```python
from build123d import *

# Parameters (mm, degrees)
SKETCH_1_W          = 30
SKETCH_1_H          = 40
SKETCH_1_W_2        = 28
SKETCH_1_H_2        = 38
EXTRUDE_1_DEPTH     = 250
SKETCH_3_R          = 2.1
CUT_EXTRUDE_1_DEPTH = 250
SKETCH_4_R          = 3.5
CUT_EXTRUDE_2_DEPTH = 250
SKETCH_5_R          = 7
CUT_EXTRUDE_3_DEPTH = 250
CUT_EXTRUDE_4_DEPTH = 20
CUT_EXTRUDE_START   = -20
SKETCH_8_R          = 3.25
CUT_EXTRUDE_7_DEPTH = 22
SKETCH_9_R          = 2
CUT_EXTRUDE_8_DEPTH = 36


with BuildPart() as part:
    # 草图1 → 凸台-拉伸1 (new body)
    with BuildSketch(Plane.XY):
        Rectangle(SKETCH_1_W, SKETCH_1_H)
        Rectangle(SKETCH_1_W_2, SKETCH_1_H_2, mode=Mode.SUBTRACT)
    extrude(amount=EXTRUDE_1_DEPTH)

    # 草图3 → 切除-拉伸1 (cut)
    with BuildSketch(Plane(origin=(0, 20, 0), x_dir=(1, 0, 0), z_dir=(0, 1, 0))):
        with Locations(Location((5, -7.5, 0), (0, 0, 270))):
            Circle(SKETCH_3_R)
        with Locations(Location((5, -22.5, 0), (0, 0, 270))):
            Circle(SKETCH_3_R)
        with Locations(Location((5, -227.5, 0), (0, 0, 90))):
            Circle(SKETCH_3_R)
        with Locations(Location((5, -242.5, 0), (0, 0, 90))):
            Circle(SKETCH_3_R)
        with Locations(Location((0, -120, 0), (0, 0, 270))):
            Circle(SKETCH_3_R)
        with Locations(Location((0, -130, 0), (0, 0, 90))):
            Circle(SKETCH_3_R)
    extrude(amount=-CUT_EXTRUDE_1_DEPTH, mode=Mode.SUBTRACT)

    # 草图4 → 切除-拉伸2 (cut)
    with BuildSketch(Plane(origin=(15, 0, 0), x_dir=(0, 0, -1), z_dir=(1, 0, 0))):
        with Locations((-222, 0)):
            Circle(SKETCH_4_R)
        with Locations((-166, 0)):
            Circle(SKETCH_4_R)
        with Locations((-84, 0)):
            Circle(SKETCH_4_R)
        with Locations((-28, 0)):
            Circle(SKETCH_4_R)
    extrude(amount=-CUT_EXTRUDE_2_DEPTH, mode=Mode.SUBTRACT)

    # 草图5 → 切除-拉伸3 (cut)
    with BuildSketch(Plane.ZY.offset(15)):
        with Locations((125, 0)):
            Circle(SKETCH_5_R)
    extrude(amount=-CUT_EXTRUDE_3_DEPTH, mode=Mode.SUBTRACT)

    # 草图6 → 切除-拉伸4 (cut)
    with BuildSketch(Plane.XZ.offset(20)):
        with BuildLine():
            Line((-4, 145), (-4, 105))
            ThreePointArc((-4, 105), (4.5, 96.5), (13, 105))
            Line((13, 105), (13, 145))
            ThreePointArc((13, 145), (4.5, 153.5), (-4, 145))
        make_face()
    extrude(amount=-CUT_EXTRUDE_4_DEPTH, mode=Mode.SUBTRACT)

    # 草图8 → 切除-拉伸7 (cut)
    with BuildSketch(Plane.ZY.offset(15).offset(CUT_EXTRUDE_START)):
        with Locations((110.150757595, -14.849242405)):
            Circle(SKETCH_8_R)
        with Locations((139.849242405, -14.849242405)):
            Circle(SKETCH_8_R)
        with Locations((110.150757595, 14.849242405)):
            Circle(SKETCH_8_R)
        with Locations((139.849242405, 14.849242405)):
            Circle(SKETCH_8_R)
    extrude(amount=-CUT_EXTRUDE_7_DEPTH, mode=Mode.SUBTRACT)

    # 草图9 → 切除-拉伸8 (cut)
    with BuildSketch(Plane(origin=(15, 0, 0), x_dir=(0, 0, -1), z_dir=(1, 0, 0))):
        with Locations((-15, 6)):
            Circle(SKETCH_9_R)
        with Locations((-15, -6)):
            Circle(SKETCH_9_R)
        with Locations((-235, -6)):
            Circle(SKETCH_9_R)
        with Locations((-235, 6)):
            Circle(SKETCH_9_R)
    extrude(amount=-CUT_EXTRUDE_8_DEPTH, mode=Mode.SUBTRACT)


solid = part.part
```
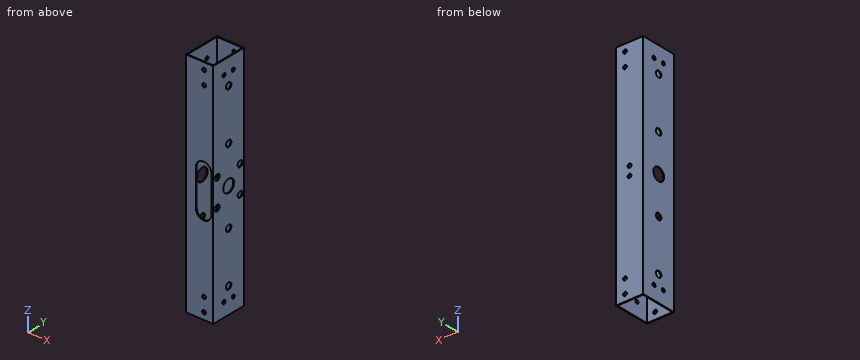
The listing builds one solid part. Answer for the finished solid, in the listing's coordinates (mm). Round coordinates to 2 decimals unless told otherwise and drop trailing zeros. Loops run counter-clockwise (first coordinate to the right, second up) from the corner with the lowest first, then second, coordinate; pieces in that order, holes last. Notation, with made-up numbers: (29.25, 21.25) - (52.25, 21.25) arc R19 ccw to (52.25, 25.25) - close; hole circle Ø5 at (11, 15.25). An arc over 180 degrees is marked (long way). Return JSON: item names as keys, results as strings. Group by question number.
1. Consider probe 1 along Y at (x, z) = (14.3, 15); probe 2 along X at (y, z) = (2, 206); probe 3 along Y at (x, z) = (-12.5, 85.5). Determine where each line is inside the solid, lowest interval first.
2. The part is cut by section D-D on x = 0. Determine the outline of the cut face in (y, z).
3. The part is cut by section B-B on z = 222. Determine the outline of the cut face in (x, y), then the cut area to 3 significant figures.
4. The part is cut by section A-A on z = 125. Determine the outline of the cut face in (x, y), then the cut area to 3 significant figures.
5. The part is cut by section C-C on x = 10.75. Determine the outline of the cut face in (y, z).
6. Each of these flat-tipped pins is pushed along its axis until it touches: P1, Ø6, axis at y = 14.85, z = 110.15, coming from the +X side; P2, Ø5.5, axis at y = 0, z = 166, coming from the +X side. Where does it stop, or does it pass through?
Resolved:
{
 "1": {"probe 1": "y = -20 to -8, -4 to 4, 8 to 20", "probe 2": "x = -15 to -14, 14 to 15", "probe 3": "y = -20 to -19, 19 to 20"},
 "2": {"outline": "(-20, 0) - (-19, 0) - (-19, 97.79) - (-20, 97.79) - close; (-20, 152.21) - (-19, 152.21) - (-19, 250) - (-20, 250) - close; (19, 0) - (20, 0) - (20, 117.9) - (19, 117.9) - close; (19, 122.1) - (20, 122.1) - (20, 127.9) - (19, 127.9) - close; (19, 132.1) - (20, 132.1) - (20, 250) - (19, 250) - close"},
 "3": {"outline": "(-15, -20) - (15, -20) - (15, -3.5) - (14, -3.5) - (14, -19) - (-14, -19) - (-14, -3.5) - (-15, -3.5) - close; (-15, 3.5) - (-14, 3.5) - (-14, 19) - (14, 19) - (14, 3.5) - (15, 3.5) - (15, 20) - (-15, 20) - close", "area": "122 mm²"},
 "4": {"outline": "(-15, -20) - (-4, -20) - (-4, -19) - (-14, -19) - (-14, -7) - (-15, -7) - close; (-15, 7) - (-14, 7) - (-14, 19) - (14, 19) - (14, 7) - (15, 7) - (15, 20) - (-15, 20) - close; (13, -20) - (15, -20) - (15, -7) - (14, -7) - (14, -19) - (13, -19) - close", "area": "91.0 mm²"},
 "5": {"outline": "(-20, 0) - (-19, 0) - (-19, 99.24) - (-20, 99.24) - close; (-20, 150.76) - (-19, 150.76) - (-19, 250) - (-20, 250) - close; (19, 0) - (20, 0) - (20, 250) - (19, 250) - close"},
 "6": {"P1": "stops at x = -14", "P2": "passes through"}
}
